from build123d import *

# Parameters (mm, degrees)
SKETCH1_R           = 3
BOSS_EXTRUDE1_DEPTH = 3
DRAFT2_ANGLE        = 1
DRAFT3_ANGLE        = 20


with BuildPart() as part:
    # Sketch1 → Boss-Extrude1 (new body)
    with BuildSketch(Plane(origin=(0, 0, 0), x_dir=(1, 0, 0), z_dir=(0, 1, 0))):
        Circle(SKETCH1_R)
    extrude(amount=BOSS_EXTRUDE1_DEPTH)

    # Draft2
    draft2_faces = [part.faces().sort_by_distance(p)[0] for p in [
        (-3, 1.5, 0),
    ]]
    draft(draft2_faces, Plane.ZX.offset(3), DRAFT2_ANGLE)

    # Draft3
    draft3_faces = [part.faces().sort_by_distance(p)[0] for p in [
        (-3.026182597, 1.5, 0),
    ]]
    draft(draft3_faces, Plane.ZX.offset(3), DRAFT3_ANGLE)


solid = part.part
Input: part model. Units: mm. Frame: model coordinates. Coordinates: 2 decimals unless noted, no trailing zeros. Order: outer loops, then holes, each group sorted by start corner. A loop starts at its lowest first (then second) coordinate and runs counter-clockwise, first axis right, second up. Notation, with made-up numbers: M 11.25,86.5 L 55.25,86.5 A28 ccw 55.25,104.5 Z; hole C 23.5,31.5 d1. An arc over 180 degrees is marked long. Write item = value, one per line. Start each with the question number.
(1) Section C-C on y = 0.95. Output: boundary loops of the cut face in (x, z).
(2) Section D-D on y = 1.55. Output: boundary loops of the cut face in (x, z).
(3) Line query: line 1 along X through (y, z) = (2.7, 0.5); line 2 along Y through (x, z) = (2, 3); line 3 along Z through (x, y) = (0.25, 0.8). Output: solid intervals per line, ascending. Write a range as [from, to].
(4) Section B-B on z = 0. Output: boundary loops of the cut face in (x, y), and give its area (3 significant figures).
(5) Section A-A on x = 0. Output: boundary loops of the cut face in (y, z).
Result set:
q1.outline = C 0,0 d7.49
q2.outline = C 0,0 d7.06
q3.line_1 = [-3.07, 3.07]
q3.line_2 = [0, 1.34]
q3.line_3 = [-3.79, 3.79]
q4.outline = M -4.09,0 L 4.09,0 L 3,3 L -3,3 Z
q4.area = 21.3 mm²
q5.outline = M 0,-4.09 L 3,-3 L 3,3 L 0,4.09 Z
